Geometry check sheet. Reference: the model listing, model coordinates, mm. Face numbers are marked on the shaded views. A direction names the side the tool comes from. Round coordinates to 2 decimals unless told otherwise and drop trailing zeros. Write each loop counter-clockwise with the first axis right and the second up, starting at its lowest first coordinate (ties: lowest second). Pieces come first, ordered by that corner, then holes. Notation, with made-up numbers: M -1,31 L 8,31 A13 ccw 8,48 Z; hole C 87.25,33 d11. An arc over 180 degrees is marked long. Put each result on its own line as item: value. Start each with the question number.
(1) Gauge pin test, flat ends, axial feed: pin 1 (9 mm diameter, centred on x = -14, y = -14.5, fed in from +Z); pin 2 (1 mm diameter, centred on y = -19.5, z = 1.5, fed in from +X); pin 3 (8.5 mm diameter, centred on x = 12.7, y = -12.7, fed in from +Z). Record the tip position at first contact, or that the pin passes through.
(2) Section check D-D on y = 4.5. Record the cut outline in (x, z), then the cut area to 3 significant figures.
(3) Tool access check on the marked faces 1 and 2. Record the directions out of +Z, -Z, +X, -X, +Y, -Y that give a thin tool (end or side, any length) a straight path to the whole face; none if there is none.
(4) Material ranges on probe 1 along Y at (x, z) = (12.7, 0.45); probe 2 along Y at (x, z) = (14.5, 6.5); probe 3 along X at (y, z) = (13, 4), recorded low to high.
(5) Section check A-A on z = 3.75. Count the separate pieces of the cut face and the enclosed holes in it, then the cut area to 3 significant figures.
(6) Mould release check, pull along X, two halves, no side actions. Record for the marked faces 3, 4 and 5: pulls with the +X half, pulls with the -X half, needs draft (parallel to the pull), parting line crosses it, or undercut.
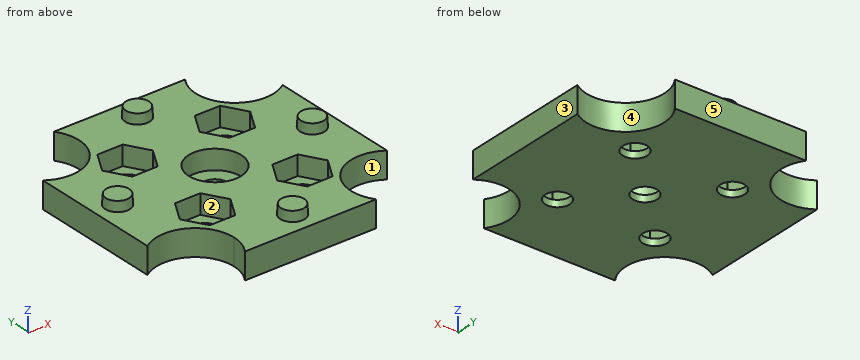
from build123d import *

# Parameters (mm, degrees)
F0_R       = 3.2004
F0_R_2     = 6.858
F1_DEPTH   = 6.8326
F2_DEPTH   = 9.3726
F3_R       = 3.2004
F3_R_2     = 6.858
F4_DEPTH   = 5.08
F5_SIZE2   = 2.53999
F5_SIZE    = 0.17779
F5_2_SIZE2 = 2.53999
F5_2_SIZE  = 0.17779
F5_3_SIZE2 = 2.53999
F5_3_SIZE  = 0.17779
F5_4_SIZE2 = 2.53999
F5_4_SIZE  = 0.17779


# Not quite as in the source:
# - a fillet or chamfer is up to 0.001 mm smaller than in the source, because OpenCascade refuses the exact size


with BuildPart() as f1:
    # F0 (on Top) → F1 (new body)
    with BuildSketch(Plane.XY):
        with BuildLine():
            ThreePointArc((-31.242, -17.0875613686), (-20.7164714157, -16.3838944106), (-15.24, -25.4))
            ThreePointArc((-15.24, -25.4), (-15.712895776, -28.4635945803), (-17.0875613686, -31.242))
            Line((-17.0875613686, -31.242), (17.0875613686, -31.242))
            ThreePointArc((17.0875613686, -31.242), (18.2157951031, -18.2157951031), (31.242, -17.0875613686))
            Line((31.242, -17.0875613686), (31.242, 17.0875613686))
            ThreePointArc((31.242, 17.0875613686), (18.2157951031, 18.2157951031), (17.0875613686, 31.242))
            Line((17.0875613686, 31.242), (-17.0875613686, 31.242))
            ThreePointArc((-17.0875613686, 31.242), (-18.2157951031, 18.2157951031), (-31.242, 17.0875613686))
            Line((-31.242, 17.0875613686), (-31.242, -17.0875613686))
        make_face()
        with Locations((0, -25.4)):
            Circle(F0_R, mode=Mode.SUBTRACT)
        with Locations((-25.4, 0)):
            Circle(F0_R, mode=Mode.SUBTRACT)
        with Locations((-12.7, -12.7)):
            Circle(F0_R, mode=Mode.SUBTRACT)
        Circle(F0_R_2, mode=Mode.SUBTRACT)
        with Locations((12.7, -12.7)):
            Circle(F0_R, mode=Mode.SUBTRACT)
        with Locations((25.4, 0)):
            Circle(F0_R, mode=Mode.SUBTRACT)
        with Locations((-12.7, 12.7)):
            Circle(F0_R, mode=Mode.SUBTRACT)
        with Locations((0, 25.4)):
            Circle(F0_R, mode=Mode.SUBTRACT)
        with Locations((12.7, 12.7)):
            Circle(F0_R, mode=Mode.SUBTRACT)
        Circle(F0_R_2)
        Circle(F0_R, mode=Mode.SUBTRACT)
    extrude(amount=F1_DEPTH)

    # F0 (on Top) → F2 (join)
    with BuildSketch(Plane.XY):
        with Locations((-25.4, 0)):
            Circle(F0_R)
        with Locations((0, -25.4)):
            Circle(F0_R)
        with Locations((25.4, 0)):
            Circle(F0_R)
        with Locations((0, 25.4)):
            Circle(F0_R)
    extrude(amount=F2_DEPTH)

    # F3 (on face) → F4 (cut)
    with BuildSketch(Plane.XY.offset(6.8326)):
        Polygon((-9.398, 6.9807682334), (-6.096, 12.7), (-9.398, 18.4192317666), (-16.002, 18.4192317666), (-19.304, 12.7), (-16.002, 6.9807682334), align=None)
        with Locations((-12.7, 12.7)):
            Circle(F3_R, mode=Mode.SUBTRACT)
        Polygon((9.398, 18.4192317666), (6.096, 12.7), (9.398, 6.9807682334), (16.002, 6.9807682334), (19.304, 12.7), (16.002, 18.4192317666), align=None)
        with Locations((12.7, 12.7)):
            Circle(F3_R, mode=Mode.SUBTRACT)
        Polygon((-9.398, -18.4192317666), (-6.096, -12.7), (-9.398, -6.9807682334), (-16.002, -6.9807682334), (-19.304, -12.7), (-16.002, -18.4192317666), align=None)
        with Locations((-12.7, -12.7)):
            Circle(F3_R, mode=Mode.SUBTRACT)
        Polygon((9.398, -6.9807682334), (6.096, -12.7), (9.398, -18.4192317666), (16.002, -18.4192317666), (19.304, -12.7), (16.002, -6.9807682334), align=None)
        with Locations((12.7, -12.7)):
            Circle(F3_R, mode=Mode.SUBTRACT)
        Circle(F3_R_2)
        Circle(F3_R, mode=Mode.SUBTRACT)
    extrude(amount=-F4_DEPTH, mode=Mode.SUBTRACT)

    # F5 (size 0.1778 and 2.54 in the source; OpenCascade refuses exactly that, so slightly less here)
    f5_edges = [f1.edges().sort_by_distance(p)[0] for p in [
        (-28.6004, 0, 9.3726),
    ]]
    f5_side = f1.faces().sort_by_distance((-25.4, 0, 9.3726))[0]
    chamfer(f5_edges, length=F5_SIZE, length2=F5_SIZE2, reference=f5_side)

    # F5#2 (size 0.1778 and 2.54 in the source; OpenCascade refuses exactly that, so slightly less here)
    f5_2_edges = [f1.edges().sort_by_distance(p)[0] for p in [
        (-3.2004, 25.4, 9.3726),
    ]]
    f5_2_side = f1.faces().sort_by_distance((0, 25.4, 9.3726))[0]
    chamfer(f5_2_edges, length=F5_2_SIZE, length2=F5_2_SIZE2, reference=f5_2_side)

    # F5#3 (size 0.1778 and 2.54 in the source; OpenCascade refuses exactly that, so slightly less here)
    f5_3_edges = [f1.edges().sort_by_distance(p)[0] for p in [
        (22.1996, 0, 9.3726),
    ]]
    f5_3_side = f1.faces().sort_by_distance((25.4, 0, 9.3726))[0]
    chamfer(f5_3_edges, length=F5_3_SIZE, length2=F5_3_SIZE2, reference=f5_3_side)

    # F5#4 (size 0.1778 and 2.54 in the source; OpenCascade refuses exactly that, so slightly less here)
    f5_4_edges = [f1.edges().sort_by_distance(p)[0] for p in [
        (-3.2004, -25.4, 9.3726),
    ]]
    f5_4_side = f1.faces().sort_by_distance((0, -25.4, 9.3726))[0]
    chamfer(f5_4_edges, length=F5_4_SIZE, length2=F5_4_SIZE2, reference=f5_4_side)


solid = f1.part
Answers follow:
1. pin 1: stops at z = 6.83
1. pin 2: stops at x = 17.51
1. pin 3: stops at z = 1.75
2. outline: M -31.24,0 L 31.24,0 L 31.24,6.83 L 5.18,6.83 L 5.18,1.75 L -5.18,1.75 L -5.18,6.83 L -31.24,6.83 Z
2. area: 374 mm^2
3. face 1: +Z, -Z
3. face 2: +Z
4. probe 1: y = -31.24 to -15.9, -9.5 to 9.5, 15.9 to 31.24
4. probe 2: y = -31.24 to -18.42, -6.98 to 6.98, 18.42 to 31.24
4. probe 3: x = -31.24 to -19.13, -6.27 to 6.27, 19.13 to 31.24
5. separate pieces: 1
5. enclosed holes: 5
5. area: 2,400 mm^2
6. face 3: pulls with the +X half
6. face 4: undercut
6. face 5: needs draft
